For this review, use the dimensioned drawing (mm, ordinates from the lowest corner) and the shaded views. A direction names the side the tool comes from. Coordinates: 2 decimals unless noted, no trailing zeros. Loops run counter-clockwise (first coordinate to the right, second up) from the corner with the lowest first, then second, coordinate; pieces in that order, holes last. Notation, with made-up numbers: M -32.75,72 L -8.75,72 A34 ccw -8.75,109 Z; hole C 24,-32 d10. An arc over 180 degrees is marked long. One line per item, written item: value.
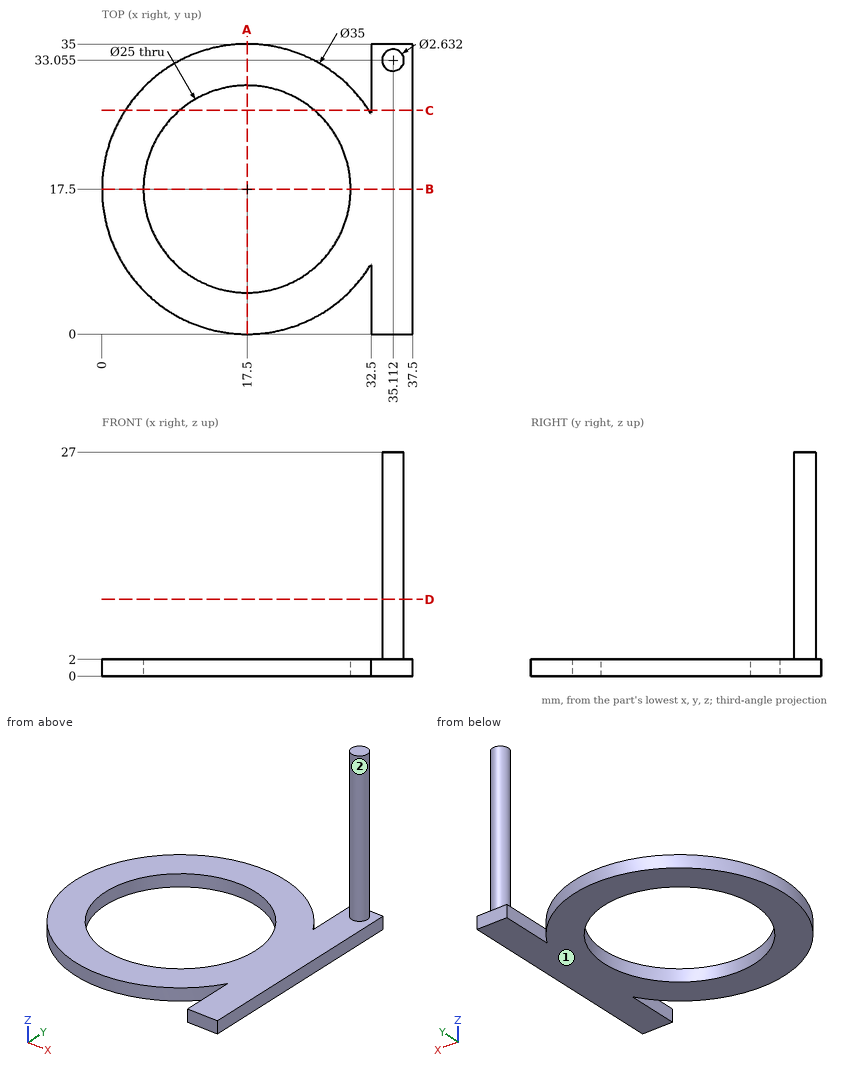
(1) We need section C-C on y = 27. State the section outline as (x, z) points, then the cut area to 3 significant figures.
Reply:
outline: M 2.8,0 L 9.38,0 L 9.38,2 L 2.8,2 Z; M 25.62,0 L 32.2,0 L 32.2,2 L 25.62,2 Z; M 32.5,0 L 37.5,0 L 37.5,2 L 32.5,2 Z
area: 36.3 mm2
(2) Tool access review of the marked faces 1 and 2: name each direction out of +Z, -Z, +X, -X, +Y, -Y from which nothing blocks a thin tool from reaching the whole face with its end or side.
Reply:
face 1: -Z, +X, -X, +Y, -Y
face 2: +Z
(3) We need section A-A on x = 17.5. State the section outline as (y, z) points.
Reply:
outline: M 0,0 L 5,0 L 5,2 L 0,2 Z; M 30,0 L 35,0 L 35,2 L 30,2 Z
(4) To check wall thickness, follow line 1 along Y through (x, z) = (17.5, 1.6); line 2 along Z through (x, y) = (34, 3); line 3 along Y through (x, z) = (2.5, 1.5) (1 decimal). State the ranges of each line that lie inside material, in increasing order. Write a range as [from, to].
Reply:
line 1: y = [0, 5], [30, 35]
line 2: z = [0, 2]
line 3: y = [8.5, 26.5]
(5) We need section D-D on z = 9.25. State the section outline as (x, y) points (1 decimal).
Reply:
outline: C 35.1,33.1 d2.6
(6) We need section B-B on y = 17.5. State the section outline as (x, z) points, then the cut area to 3 significant figures.
Reply:
outline: M 0,0 L 5,0 L 5,2 L 0,2 Z; M 30,0 L 37.5,0 L 37.5,2 L 30,2 Z
area: 25.0 mm2
(7) Insertion check: pin 1 (12 mm diameter, centred on x = 22, y = 20, fed in from -Z); pin 2 (1 mm diameter, centred on y = 6, z = 1.5, fed in from -X); pin 3 (0.6 mm diameter, centred on y = 32.5, z = 1.5, fed in from -X) (1 decimal); pin 4 (6 mm diameter, centred on y = 27.5, z = 4, fed in from -X). Each pin has a flat end and moves straight along its axis. Give the tip position at first contact, or say it passes through.
Reply:
pin 1: passes through
pin 2: stops at x = 3.89
pin 3: stops at x = 8
pin 4: stops at x = 1.82
